from build123d import *

# Parameters (mm, degrees)
SKETCH1_W                                    = 45
SKETCH1_H                                    = 25
BOSS_EXTRUDE1_DEPTH                          = 15
HOLE1_D                                      = 6.8
HOLE1_DEPTH                                  = 10
CBORE_FOR_M5_HEX_SOCKET_HEAD_CAP_SCR_2_COUNT = 2
CBORE_FOR_M5_HEX_SOCKET_HEAD_CAP_SCR_2_PITCH = 30
FILLET1_R                                    = 2
CHAMFER1_SIZE                                = 0.6


with BuildPart() as part:
    # Sketch1 → Boss-Extrude1 (new body)
    with BuildSketch(Plane(origin=(0, 0, 0), x_dir=(1, 0, 0), z_dir=(0, 1, 0))):
        Rectangle(SKETCH1_W, SKETCH1_H)
    extrude(amount=BOSS_EXTRUDE1_DEPTH)

    # Hole1
    with Locations(Plane(origin=(0, 15, 0), x_dir=(1, 0, 0), z_dir=(0, 1, 0))):
        with Locations((0, 0)):
            Hole(HOLE1_D / 2, depth=HOLE1_DEPTH)

    # Sketch7 → CBORE for M5 Hex Socket Head Cap Screw1 (revolve, cut)
    with BuildSketch(Plane(origin=(15, 15, 0), x_dir=(0, 0, 1), z_dir=(1, 0, 0))):
        Polygon((0, 0), (0, 15), (2.75, 15), (2.75, 5.4), (5, 5.4), (5, 0.025), (5.025, 0), align=None)
    cbore_for_m5_hex_socket_head_cap_screw1 = revolve(axis=Axis((15, 21.35, 0), (0, -1, 0)), mode=Mode.SUBTRACT)

    # CBORE for M5 Hex Socket Head Cap Scr 2: CBORE for M5 Hex Socket Head Cap Screw1 ×2
    with Locations(*[(-i * CBORE_FOR_M5_HEX_SOCKET_HEAD_CAP_SCR_2_PITCH, 0, 0) for i in range(1, CBORE_FOR_M5_HEX_SOCKET_HEAD_CAP_SCR_2_COUNT)]):
        add(cbore_for_m5_hex_socket_head_cap_screw1, mode=Mode.SUBTRACT)

    # Fillet1
    fillet1_edges = [part.edges().sort_by_distance(p)[0] for p in [
        (-22.5, 7.5, -12.5),
        (22.5, 7.5, -12.5),
        (22.5, 7.5, 12.5),
        (-22.5, 7.5, 12.5),
    ]]
    fillet(fillet1_edges, radius=FILLET1_R)

    # Chamfer1
    chamfer1_edges = [part.edges().sort_by_distance(p)[0] for p in [
        (3.4, 15, 0),
        (15, 0, -2.75),
        (-15, 0, -2.75),
        (-22.5, 0, 0),
        (-22.5, 15, 0),
        (0, 0, -12.5),
        (22.5, 0, 0),
        (0, 0, 12.5),
        (21.914213562, 0, 11.914213562),
        (21.914213562, 0, -11.914213562),
        (-21.914213562, 0, 11.914213562),
        (-21.914213562, 0, -11.914213562),
        (0, 15, -12.5),
        (0, 15, 12.5),
        (22.5, 15, 0),
        (21.914213562, 15, 11.914213562),
        (21.914213562, 15, -11.914213562),
        (-21.914213562, 15, 11.914213562),
        (-21.914213562, 15, -11.914213562),
    ]]
    chamfer(chamfer1_edges, length=CHAMFER1_SIZE)


solid = part.part
Verification items for the finished model (mm, model axes). A direction names the side the tool comes from. Coordinates: 2 decimals unless noted, no trailing zeros. Order: outer loops, then holes, each group sorted by start corner. A loop starts at its lowest first (then second) coordinate and runs counter-clockwise, first axis right, second up.
Item 1: Section check A-A, the plane x = 15. Enter the section's corners in (y, z) (3 decimals).
Filled in:
outline: (0, -11.9) - (0.6, -12.5) - (14.4, -12.5) - (15, -11.9) - (15, -5.025) - (14.975, -5) - (9.6, -5) - (9.6, -2.75) - (0.6, -2.75) - (0, -3.35) - close; (0, 3.35) - (0.6, 2.75) - (9.6, 2.75) - (9.6, 5) - (14.975, 5) - (15, 5.025) - (15, 11.9) - (14.4, 12.5) - (0.6, 12.5) - (0, 11.9) - close
Item 2: Release check for a two-part mould opening along X. For faces 1 (the face through (17.2, 9.6, -2.2)), 2 (the face through (0, 7, -12.5)), 3 (the face through (-21.639, 0.229, 11.665)) record: +X half, -X half, draft (parallel to the pull), parting line (faces both ways), or undercut.
Filled in:
face 1: undercut
face 2: draft
face 3: -X half
Item 3: Access from +Z, -Z, +X, -X, +Y, -Y to the whole of each face (thin tool, end or side, straight path). Record for faces 4 (the face through (19.88, 12.33, -1.08)), 5 (the face through (21.9, 7.6, 11.93)).
Filled in:
face 4: +Y
face 5: +Z, +X, +Y, -Y
Item 4: Section check C-C, the plane z = 0. Give the number of separate pieces and of enclosed holes in the cut face, then the cut area to 3 significant figures.
Filled in:
separate pieces: 3
enclosed holes: 0
area: 392 mm2
Item 5: Section check D-D, the plane x = 0. Enter the section's corners in (y, z).
Filled in:
outline: (0, -11.9) - (0.6, -12.5) - (14.4, -12.5) - (15, -11.9) - (15, -4) - (14.4, -3.4) - (5, -3.4) - (5, 3.4) - (14.4, 3.4) - (15, 4) - (15, 11.9) - (14.4, 12.5) - (0.6, 12.5) - (0, 11.9) - close
Item 6: Section check B-B, the plane y = 13.25. Enter the section's corners in (x, z).
Filled in:
outline: (-22.5, -10.5) arc R2 ccw to (-20.5, -12.5) - (20.5, -12.5) arc R2 ccw to (22.5, -10.5) - (22.5, 10.5) arc R2 ccw to (20.5, 12.5) - (-20.5, 12.5) arc R2 ccw to (-22.5, 10.5) - close; hole circle Ø10 at (-15, 0); hole circle Ø6.8 at (0, 0); hole circle Ø10 at (15, 0)
Item 7: Material ranges on L1, parallel to X at y = 4.75, z = 0; L2, parallel to X at y = 6.75, z = 0; L3, parallel to Z at x = 15, y = 11.85, recorded low to high.
Filled in:
L1: x = -22.5 to -17.75, -12.25 to 12.25, 17.75 to 22.5
L2: x = -22.5 to -17.75, -12.25 to -3.4, 3.4 to 12.25, 17.75 to 22.5
L3: z = -12.5 to -5, 5 to 12.5
Item 8: Depth check by flat-ended pin: pin 1 (8 mm diameter, centred on x = -13.5, z = 2.5, fed in from +Y); pin 2 (6 mm diameter, centred on x = 15, z = 0, fed in from +Y); pin 3 (3.5 mm diameter, centred on x = 1, z = 1.5, fed in from +Y). Enter the tip coordinate at first touch or a pass-through.
Filled in:
pin 1: stops at y = 15
pin 2: stops at y = 9.6
pin 3: stops at y = 14.55
